Build history of the part. All positions in model axes, mm. Face numbers are marked on the shaded views. A direction names the side the tool comes from. Round coordinates to 2 decimals unless told otherwise and drop trailing zeros. Loops run counter-clockwise (first coordinate to the right, second up) from the corner with the lowest first, then second, coordinate; pieces in that order, holes last.
from build123d import *

# Parameters (mm, degrees)
ESQUISSE1_W             = 22
ESQUISSE1_H             = 7
ESQUISSE1_R             = 1.5
ESQUISSE1_H_2           = 10
BOSS_EXTRU_1_DEPTH      = 8
ESQUISSE1_3_W           = 22
ESQUISSE1_3_H           = 10
BOSS_EXTRU_2_DEPTH      = 15
ESQUISSE2_W             = 22
ESQUISSE2_H             = 7.5
BOSS_EXTRU_3_DEPTH      = 60
ESQUISSE3_W             = 22
ESQUISSE3_H             = 10
BOSS_EXTRU_4_DEPTH      = 54
ESQUISSE4_W             = 52
ESQUISSE4_H             = 33
BOSS_EXTRU_5_DEPTH      = 5
ESQUISSE6_R             = 2
ENL_V_MAT_EXTRU_1_DEPTH = 5


with BuildPart() as part:
    # Esquisse1 → Boss.-Extru.1 (new body)
    # profile 1 of 3: a face of its own
    with BuildSketch(Plane.XY):
        with Locations((11, 20.5)):
            Rectangle(ESQUISSE1_W, ESQUISSE1_H)
        with Locations((3, 21)):
            Circle(ESQUISSE1_R, mode=Mode.SUBTRACT)
        with Locations((19, 21)):
            Circle(ESQUISSE1_R, mode=Mode.SUBTRACT)
    # profile 2 of 3: a face of its own
    with BuildSketch(Plane.XY):
        with Locations((11, 12)):
            Rectangle(ESQUISSE1_W, ESQUISSE1_H_2)
    # profile 3 of 3: a face of its own
    with BuildSketch(Plane.XY):
        with Locations((11, 3.5)):
            Rectangle(ESQUISSE1_W, ESQUISSE1_H)
        with Locations((3, 3)):
            Circle(ESQUISSE1_R, mode=Mode.SUBTRACT)
        with Locations((19, 3)):
            Circle(ESQUISSE1_R, mode=Mode.SUBTRACT)
    extrude(amount=BOSS_EXTRU_1_DEPTH)

    # Esquisse1_3 → Boss.-Extru.2 (add)
    with BuildSketch(Plane.XY):
        with Locations((11, 12)):
            Rectangle(ESQUISSE1_3_W, ESQUISSE1_3_H)
    extrude(amount=-BOSS_EXTRU_2_DEPTH)

    # Esquisse2 → Boss.-Extru.3 (add)
    with BuildSketch(Plane.XZ.offset(-7)):
        with Locations((11, -11.25)):
            Rectangle(ESQUISSE2_W, ESQUISSE2_H)
    extrude(amount=BOSS_EXTRU_3_DEPTH)

    # Esquisse3 → Boss.-Extru.4 (add)
    with BuildSketch(Plane(origin=(0, 0, -15), x_dir=(-1, 0, 0), z_dir=(0, 0, -1))):
        with Locations((-11, -48)):
            Rectangle(ESQUISSE3_W, ESQUISSE3_H)
    extrude(amount=BOSS_EXTRU_4_DEPTH)

    # Esquisse4 → Boss.-Extru.5 (add)
    with BuildSketch(Plane(origin=(0, 0, -69), x_dir=(-1, 0, 0), z_dir=(0, 0, -1))):
        with Locations((-11, -48)):
            Rectangle(ESQUISSE4_W, ESQUISSE4_H)
    extrude(amount=-BOSS_EXTRU_5_DEPTH)

    # Esquisse6 → Enl_v. mat.-Extru.1 (cut)
    with BuildSketch(Plane(origin=(0, 0, -69), x_dir=(-1, 0, 0), z_dir=(0, 0, -1))):
        with Locations((-25, -34.75)):
            Circle(ESQUISSE6_R)
        with Locations((-25, -61.5)):
            Circle(ESQUISSE6_R)
        with Locations((3, -34.75)):
            Circle(ESQUISSE6_R)
        with Locations((3, -61.5)):
            Circle(ESQUISSE6_R)
    extrude(amount=-ENL_V_MAT_EXTRU_1_DEPTH, mode=Mode.SUBTRACT)


solid = part.part
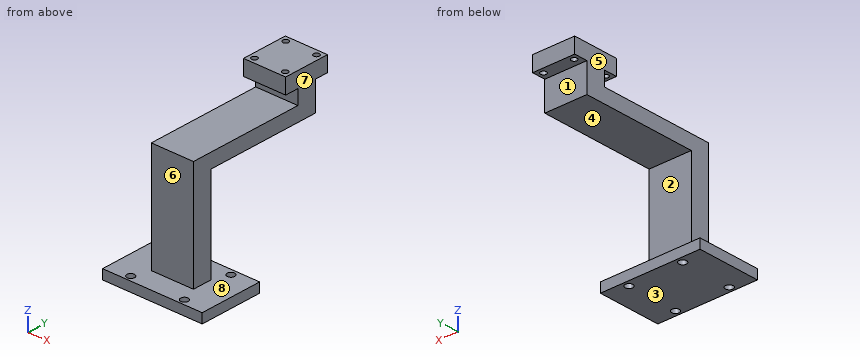
(1) Slice it at A-A on y = -41. List the corners of the cut face in (x, z).
Responses:
outline: (-15, -69) - (37, -69) - (37, -64) - (-15, -64) - close; (0, -15) - (22, -15) - (22, -7.5) - (0, -7.5) - close
(2) Slice it at B-B on x = -3. List the corners of the cut face in (y, z), plus the area to 3 significant figures.
Responses:
outline: (-64.5, -69) - (-63.5, -69) - (-63.5, -64) - (-64.5, -64) - close; (-59.5, -69) - (-36.75, -69) - (-36.75, -64) - (-59.5, -64) - close; (-32.75, -69) - (-31.5, -69) - (-31.5, -64) - (-32.75, -64) - close
area: 125 mm2
(3) Probe line 1 (Y direction, x = 25, z = -66); line 2 (X direction, y = -34, z = -66); line 3 (Z direction, x = 17, y = -23). List the from-to ranges inside material, lowest first.
Responses:
line 1: y = -64.5 to -63.5, -59.5 to -36.75, -32.75 to -31.5
line 2: x = -15 to -4.85, -1.15 to 23.15, 26.85 to 37
line 3: z = -15 to -7.5
(4) Pin check, flat tips, straight feed: P1, Ø6.5, axis at x = -3, y = -61.5, coming from the +Z side; P2, Ø2.5, axis at x = 3, y = 3, coming from the +Z side; P3, Ø2, axis at y = -46, z = -28, coming from the +X side. Stop position of each tip, or through.
Responses:
P1: stops at z = -64
P2: stops at z = -7.5
P3: stops at x = 22
(5) Pull direction Z, two halves, no side cores. Call the marked faces 1, 2 and 3: +Z half, -Z half, draft (parallel to the pull), parting line (faces both ways), or undercut.
Responses:
face 1: draft
face 2: undercut
face 3: -Z half
(6) Slice it at C-C on y = 3. List the corners of the cut face in (x, z), plus the area to 3 significant figures.
Responses:
outline: (0, -15) - (22, -15) - (22, -7.5) - (0, -7.5) - close; (0, 0) - (1.5, 0) - (1.5, 8) - (0, 8) - close; (4.5, 0) - (17.5, 0) - (17.5, 8) - (4.5, 8) - close; (20.5, 0) - (22, 0) - (22, 8) - (20.5, 8) - close
area: 293 mm2
(7) Slice it at D-D on x = 12. List the corners of the cut face in (y, z), plus the area to 3 significant figures.
Responses:
outline: (-64.5, -69) - (-31.5, -69) - (-31.5, -64) - (-43, -64) - (-43, -15) - (17, -15) - (17, 0) - (24, 0) - (24, 8) - (0, 8) - (0, 0) - (7, 0) - (7, -7.5) - (-53, -7.5) - (-53, -64) - (-64.5, -64) - close
area: 1,450 mm2
(8) Which spindle directions (+Z, -Z, +X, -X, +Y, -Y) get a long thin tool onto all of the face, cutting with end or side? Do the marked faces 4, 5, 6, 7 and 8. Say none if no direction does.
Responses:
face 4: +X, -X, +Y
face 5: +Z, -X, +Y, -Y
face 6: +Z, +X, -X, -Y
face 7: +Z, +X, +Y, -Y
face 8: none
